```python
from build123d import *

# Parameters (mm, degrees)
BOSS_EXTRUDE2_DEPTH = 5
BOSS_EXTRUDE3_DEPTH = 2
SKETCH8_W           = 2.5
SKETCH8_H           = 7
BOSS_EXTRUDE4_DEPTH = 5.96
SKETCH10_W          = 7
SKETCH10_H          = 2.49
BOSS_EXTRUDE5_DEPTH = 3
SKETCH11_W          = 7
SKETCH11_H          = 2.49
BOSS_EXTRUDE6_DEPTH = 5
SKETCH12_W          = 17
SKETCH12_H          = 2.5
BOSS_EXTRUDE7_DEPTH = 10
CUT_EXTRUDE7_REACH  = 39.855
SKETCH14_W          = 13
SKETCH14_H          = 8.75
SKETCH16_W          = 17
SKETCH16_H          = 1.25
BOSS_EXTRUDE8_DEPTH = 9.5
CUT_EXTRUDE8_REACH  = 32.06
SKETCH17_R          = 3.51
FILLET7_R           = 2
FILLET8_R           = 5
FILLET9_R           = 5
CHAMFER1_SIZE       = 2
CHAMFER2_SIZE       = 2
FILLET11_R          = 2
FILLET12_R          = 2
FILLET13_R          = 2
FILLET14_R          = 2
FILLET16_R          = 2
CHAMFER3_SIZE       = 0.5


with BuildPart() as part:
    # Sketch2 → Boss-Extrude2 (new body)
    with BuildSketch(Plane.XY):
        Polygon((15.905331571, 19.450007488), (-15.905331571, 19.450007488), (-16.612438353, 18.742900707), (-18.380205305, 20.51066766), (-16.54629868, 22.344574285), (16.54629868, 22.344574285), (18.3802029, 20.510670065), (16.610591633, 18.741058798), align=None)
    extrude(amount=BOSS_EXTRUDE2_DEPTH)

    # Sketch2_2 → Boss-Extrude3 (add)
    with BuildSketch(Plane.XY):
        Polygon((15.905331571, 19.450007488), (-15.905331571, 19.450007488), (-16.612438353, 18.742900707), (-18.380205305, 20.51066766), (-16.54629868, 22.344574285), (16.54629868, 22.344574285), (18.3802029, 20.510670065), (16.610591633, 18.741058798), align=None)
    extrude(amount=-BOSS_EXTRUDE3_DEPTH)

    # Sketch8 → Boss-Extrude4 (add)
    with BuildSketch(Plane(origin=(0, 19.450007488, 0), x_dir=(-1, 0, 0), z_dir=(0, -1, 0))):
        with Locations((11.1, -1.5)):
            Rectangle(SKETCH8_W, SKETCH8_H)
        with Locations((-11.1, -1.5)):
            Rectangle(SKETCH8_W, SKETCH8_H)
    extrude(amount=BOSS_EXTRUDE4_DEPTH)

    # Sketch10 → Boss-Extrude5 (add)
    with BuildSketch(Plane.ZY.offset(-9.85)):
        with Locations((1.5, 14.735007488)):
            Rectangle(SKETCH10_W, SKETCH10_H)
    extrude(amount=BOSS_EXTRUDE5_DEPTH)

    # Sketch11 → Boss-Extrude6 (add)
    with BuildSketch(Plane(origin=(-9.85, 0, 0), x_dir=(0, 0, -1), z_dir=(1, 0, 0))):
        with Locations((-1.5, 14.735007488)):
            Rectangle(SKETCH11_W, SKETCH11_H)
    extrude(amount=BOSS_EXTRUDE6_DEPTH)

    # Sketch12 → Boss-Extrude7 (add)
    with BuildSketch(Plane(origin=(0, 22.344574285, 0), x_dir=(1, 0, 0), z_dir=(0, 1, 0))):
        with Locations((0, -3.75)):
            Rectangle(SKETCH12_W, SKETCH12_H)
    extrude(amount=BOSS_EXTRUDE7_DEPTH)

    # Sketch14 → Cut-Extrude7 (cut, up to next)
    with BuildSketch(Plane.XY.offset(5), mode=Mode.PRIVATE) as cut_extrude7_sk1:
        with Locations((0, 26.719574285)):
            Rectangle(SKETCH14_W, SKETCH14_H)
    cut_extrude7_tool1 = extrude(cut_extrude7_sk1.sketch, amount=-CUT_EXTRUDE7_REACH, mode=Mode.PRIVATE) & part.part
    add(cut_extrude7_tool1.solids().sort_by_distance((0, 26.719574, 5))[0], mode=Mode.SUBTRACT)

    # Sketch16 → Boss-Extrude8 (add)
    with BuildSketch(Plane.XY.offset(5)):
        with Locations((0, 31.719574285)):
            Rectangle(SKETCH16_W, SKETCH16_H)
    extrude(amount=BOSS_EXTRUDE8_DEPTH)

    # Sketch17 → Cut-Extrude8 (cut, up to next)
    with BuildSketch(Plane(origin=(0, 32.344574285, 0), x_dir=(1, 0, 0), z_dir=(0, 1, 0)), mode=Mode.PRIVATE) as cut_extrude8_sk1:
        with Locations(Location((0, -9, 0), (0, 0, 270))):
            Circle(SKETCH17_R)
    cut_extrude8_tool1 = extrude(cut_extrude8_sk1.sketch, amount=-CUT_EXTRUDE8_REACH, mode=Mode.PRIVATE) & part.part
    add(cut_extrude8_tool1.solids().sort_by_distance((0, 32.344574, 9))[0], mode=Mode.SUBTRACT)

    # Fillet7
    fillet7_edges = [part.edges().sort_by_distance(p)[0] for p in [
        (7.5, 31.094574285, 5),
    ]]
    fillet(fillet7_edges, radius=FILLET7_R)

    # Fillet8
    fillet8_edges = [part.edges().sort_by_distance(p)[0] for p in [
        (8.5, 31.719574285, 14.5),
    ]]
    fillet(fillet8_edges, radius=FILLET8_R)

    # Fillet9
    fillet9_edges = [part.edges().sort_by_distance(p)[0] for p in [
        (-8.5, 31.719574285, 14.5),
    ]]
    fillet(fillet9_edges, radius=FILLET9_R)

    # Chamfer1
    chamfer1_edges = [part.edges().sort_by_distance(p)[0] for p in [
        (-12.35, 13.490007488, 1.5),
    ]]
    chamfer(chamfer1_edges, length=CHAMFER1_SIZE)

    # Chamfer2
    chamfer2_edges = [part.edges().sort_by_distance(p)[0] for p in [
        (12.35, 13.490007488, 1.5),
    ]]
    chamfer(chamfer2_edges, length=CHAMFER2_SIZE)

    # Fillet11
    fillet11_edges = [part.edges().sort_by_distance(p)[0] for p in [
        (-8.5, 22.344574285, 3.75),
    ]]
    fillet(fillet11_edges, radius=FILLET11_R)

    # Fillet12
    fillet12_edges = [part.edges().sort_by_distance(p)[0] for p in [
        (8.5, 22.344574285, 3.75),
    ]]
    fillet(fillet12_edges, radius=FILLET12_R)

    # Fillet13
    fillet13_edges = [part.edges().sort_by_distance(p)[0] for p in [
        (8.5, 22.344574285, 2.5),
    ]]
    fillet(fillet13_edges, radius=FILLET13_R)

    # Fillet14
    fillet14_edges = [part.edges().sort_by_distance(p)[0] for p in [
        (-8.5, 22.344574285, 2.5),
    ]]
    fillet(fillet14_edges, radius=FILLET14_R)

    # Fillet16
    fillet16_edges = [part.edges().sort_by_distance(p)[0] for p in [
        (-7.5, 31.094574285, 5),
    ]]
    fillet(fillet16_edges, radius=FILLET16_R)

    # Chamfer3
    chamfer3_edges = [part.edges().sort_by_distance(p)[0] for p in [
        (0, 32.344574285, 5.49),
    ]]
    chamfer(chamfer3_edges, length=CHAMFER3_SIZE)


solid = part.part
```
Work out the finished part from the listing and answer in its coordinate system (mm). A direction names the side the tool comes from. Round coordinates to 2 decimals unless told otherwise and drop trailing zeros. Order: outer loops, then holes, each group sorted by start corner. A loop starts at its lowest first (then second) coordinate and runs counter-clockwise, first axis right, second up.
Q1. A cutting plane is placed at A-A, the plane y = 25. Determine the outline of the cut face in (x, z), then the cut area to 3 significant figures.
Solution:
outline: (-8.5, 2.5) - (-6.5, 2.5) - (-6.5, 5) - (-8.5, 5) - close; (6.5, 2.5) - (8.5, 2.5) - (8.5, 5) - (6.5, 5) - close
area: 10.0 mm2
Q2. A cutting plane is placed at B-B, the plane z = 9. Determine the outline of the cut face in (x, y), then the cut area to 3 significant figures.
Solution:
outline: (-8.5, 31.09) - (-3.51, 31.09) - (-3.51, 31.84) - (-4.01, 32.34) - (-8.5, 32.34) - close; (3.51, 31.09) - (8.5, 31.09) - (8.5, 32.34) - (4.01, 32.34) - (3.51, 31.84) - close
area: 12.2 mm2
Q3. A cutting plane is placed at C-C, the plane x = 0. Determine the outline of the cut face in (y, z).
Solution:
outline: (19.45, -2) - (22.34, -2) - (22.34, 5) - (19.45, 5) - close; (31.09, 2.5) - (32.34, 2.5) - (32.34, 4.99) - (31.84, 5.49) - (31.09, 5.49) - close; (31.09, 12.51) - (31.84, 12.51) - (32.34, 13.01) - (32.34, 14.5) - (31.09, 14.5) - close
Q4. Find the intervals of material crossed by line 1 along X through (y, z) = (28, 3); line 2 along Y through (x, z) = (-6, 3.25); line 3 along X through (y, z) = (17.75, 1), in increasing order.
Solution:
line 1: x = -8.5 to -6.5, 6.5 to 8.5
line 2: y = 13.49 to 15.98, 19.45 to 22.34, 31.09 to 32.34
line 3: x = -12.35 to -9.85, 9.85 to 12.35
Q5. The mould has two halves that part along X. Classify faces 1 (the flat face through (-4.85, 15, 2)), 2 (the flat face through (-8.5, 29, 4)), 3 (the flat face through (14, 19.45, 2)), 4 (the flat face through (0, 32, 2.5)): pulls with the +X half, pulls with the -X half, needs draft (parallel to the pull), parting line crosses it, or undercut.
Solution:
face 1: undercut
face 2: pulls with the -X half
face 3: undercut
face 4: needs draft
Q6. A tool of negligible diameter and unlimited length cuts with its end or side. For faces 5 (the flat face through (1.8, 31.095, 5.7)), 6 (the flat face through (-7, 15.98, 2)), 7 (the flat face through (12.35, 17, 2)), 8 (the flat face through (0, 21, 5)), from which of +Z, -Z, +X, -X, +Y, -Y can it reach the whole face along a straight path? Write none if from no direction.
Solution:
face 5: +Z
face 6: +Z, -Z
face 7: +Z, -Z, -Y
face 8: +Z, +X, -X, -Y
Q7. A cutting plane is placed at D-D, the plane y = 17.25. Determine the outline of the cut face in (x, z), then the cut area to 3 significant figures.
Solution:
outline: (-12.35, -2) - (-9.85, -2) - (-9.85, 5) - (-12.35, 5) - close; (9.85, -2) - (12.35, -2) - (12.35, 5) - (9.85, 5) - close
area: 35.0 mm2
Q8. Given pin 1 Ø8 at (x, y) = (13, 16.5) entering from +Z; pin 2 Ø2.5 at (x, y) = (1.5, 30) entering from -Z; pin 3 Ø2.5 at (y, z) = (15, 2.5) entering from -X, each flat-ended and moving along its own axis, determine where each tip first touches the part or whether it passes through.
Solution:
pin 1: stops at z = 5
pin 2: stops at z = 2.5
pin 3: stops at x = -12.35
